Part print with two shaded views. Sizes in mm from the minimum x, y, z corner. A direction names the side the tool comes from. Round coordinates to 2 decimals unless told otherwise and drop trailing zeros. Loops run counter-clockwise (first coordinate to the right, second up) from the corner with the lowest first, then second, coordinate; pieces in that order, holes last. Notation, with made-up numbers: M 80.25,45.5 L 139.25,45.5 A22 cw 139.25,83.5 Z; hole C 74,26 d10. An arc over 180 degrees is marked long. Use a Markdown table: item, result. Add a question column.
Item 1: Wall check: L1, parallel to X at y = 5, z = 11.75; L2, parallel to Z at x = 3.5, y = 14.25; L3, parallel to Y at x = 5, z = 12.5. Give the ranges that are in metal, low to high. Write a range as from..to.
Item 2: Pin check, flat tips, straight feed: P1, Ø2, axis at x = 2.5, z = 11.5, coming from the -Y side; P2, Ø4, axis at x = 5, y = 4.5, coming from the +Z side; P3, Ø1, axis at y = 13, z = 13.5, coming from the -X side. Stop position of each tip, or through.
Item 3: Saw through at C-C on x = 6.5. Write the cut outline in (y, z), then the cut area to 3 significant figures.
Item 4: Saw through at B-B on y = 10. Write the cut outline in (x, z) (1 decimal), then the cut area to 3 significant figures.
Item 5: Saw through at D-D on y = 12. Write the cut outline in (x, z) (3 decimals).
Item 6: Saw through at A-A on z = 15.25. Write the cut outline in (x, y) (3 decimals), then the cut area to 3 significant figures.
Item 7: Tool access for the marked faces 1, 2, 3 and 4: list every direction of +Z, -Z, +X, -X, +Y, -Y with a clear straight run to the whole face (end or side of a thin tool).
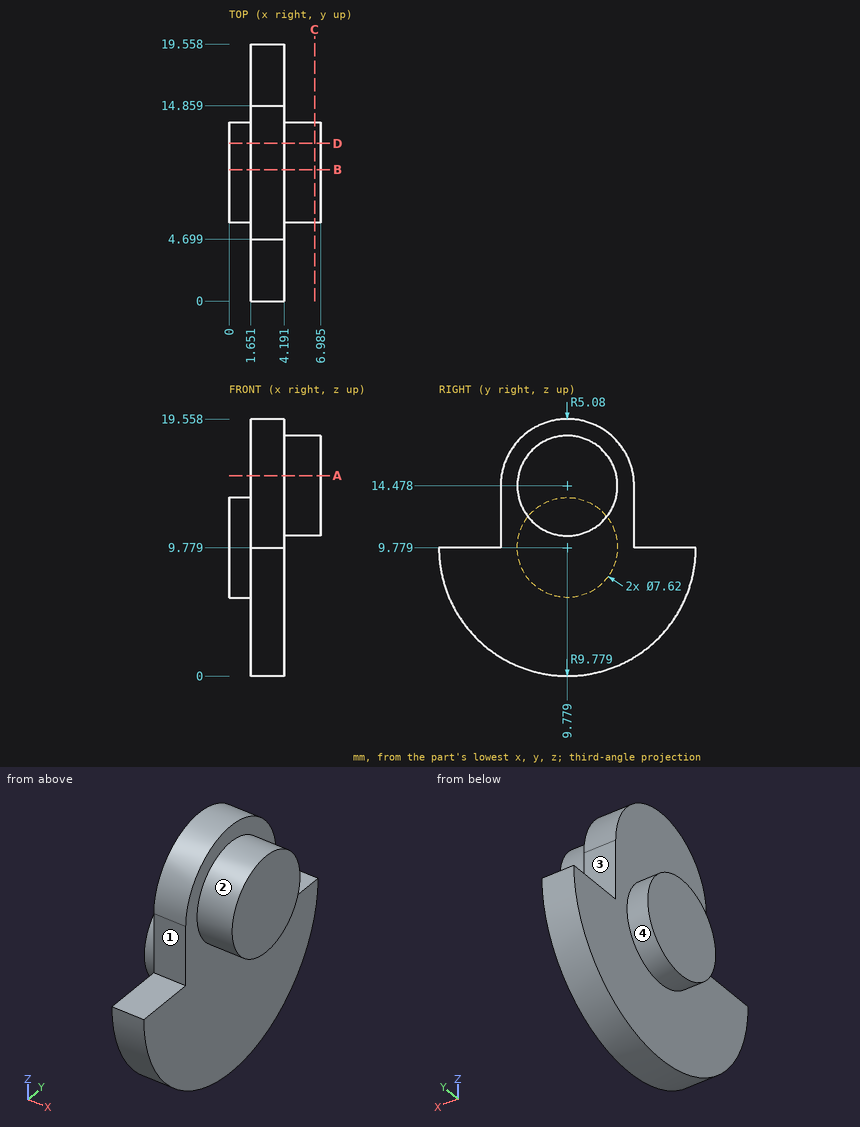
Entries:
| question | item | result |
|---|---|---|
| 1 | L1 | 1.65..4.19 |
| 1 | L2 | 1.08..16.89 |
| 1 | L3 | 6.52..13.04 |
| 2 | P1 | y = 4.7 |
| 2 | P2 | z = 18.21 |
| 2 | P3 | x = 1.65 |
| 3 | outline | C 9.78,14.48 d7.62 |
| 3 | area | 45.6 mm2 |
| 4 | outline | M 0,6 L 1.7,6 L 1.7,0 L 4.2,0 L 4.2,10.7 L 7,10.7 L 7,18.3 L 4.2,18.3 L 4.2,19.6 L 1.7,19.6 L 1.7,13.6 L 0,13.6 Z |
| 4 | area | 83.5 mm2 |
| 5 | outline | M 0,6.683 L 1.651,6.683 L 1.651,0.256 L 4.191,0.256 L 4.191,11.382 L 6.985,11.382 L 6.985,17.574 L 4.191,17.574 L 4.191,19.047 L 1.651,19.047 L 1.651,12.875 L 0,12.875 Z |
| 6 | outline | M 1.651,4.758 L 4.191,4.758 L 4.191,6.048 L 6.985,6.048 L 6.985,13.51 L 4.191,13.51 L 4.191,14.8 L 1.651,14.8 Z |
| 6 | area | 46.4 mm2 |
| 7 | face 1 | +Z, +X, -X, -Y |
| 7 | face 2 | +X |
| 7 | face 3 | +Z, +X, -X, +Y |
| 7 | face 4 | -X |
